```python
from build123d import *

# Parameters (mm, degrees)
SKETCH1_R           = 1.75
SKETCH1_R_2         = 1.925
BOSS_EXTRUDE1_DEPTH = 15
CUT_EXTRUDE1_DEPTH  = 8
SKETCH5_W           = 11
SKETCH5_H           = 33.5
CUT_EXTRUDE6_DEPTH  = 4
SKETCH8_R           = 1.75
CUT_EXTRUDE9_DEPTH  = 14
FILLET1_R           = 1.75
FILLET2_R           = 1
FILLET3_R           = 0.5
FILLET4_R           = 1.5


with BuildPart() as part:
    # Sketch1 → Boss-Extrude1 (new body)
    with BuildSketch(Plane.XY):
        with BuildLine():
            Line((-19, 16.75), (19, 16.75))
            Line((19, 16.75), (22.75, 16.75))
            Line((22.75, 16.75), (22.75, 13))
            ThreePointArc((22.75, 13), (22.193718688, 11.034634654), (20.689914163, 9.652360515))
            ThreePointArc((20.689914163, 9.652360515), (14.75, 0), (20.689914163, -9.652360515))
            ThreePointArc((20.689914163, -9.652360515), (22.193718688, -11.034634654), (22.75, -13))
            Line((22.75, -13), (22.75, -16.75))
            Line((22.75, -16.75), (19, -16.75))
            Line((19, -16.75), (-19, -16.75))
            Line((-19, -16.75), (-22.75, -16.75))
            Line((-22.75, -16.75), (-22.75, -13))
            ThreePointArc((-22.75, -13), (-22.193718688, -11.034634654), (-20.689914163, -9.652360515))
            ThreePointArc((-20.689914163, -9.652360515), (-14.75, 0), (-20.689914163, 9.652360515))
            ThreePointArc((-20.689914163, 9.652360515), (-22.193718688, 11.034634654), (-22.75, 13))
            Line((-22.75, 13), (-22.75, 16.75))
            Line((-22.75, 16.75), (-19, 16.75))
        make_face()
        with Locations((-10, -9.5)):
            Circle(SKETCH1_R, mode=Mode.SUBTRACT)
        with Locations((10, -9.5)):
            Circle(SKETCH1_R, mode=Mode.SUBTRACT)
        with Locations((19, 13)):
            Circle(SKETCH1_R_2, mode=Mode.SUBTRACT)
        with Locations((-19, 13)):
            Circle(SKETCH1_R_2, mode=Mode.SUBTRACT)
        with Locations((-19, -13)):
            Circle(SKETCH1_R_2, mode=Mode.SUBTRACT)
        with Locations((19, -13)):
            Circle(SKETCH1_R_2, mode=Mode.SUBTRACT)
        with Locations((-11, 0)):
            Circle(SKETCH1_R_2, mode=Mode.SUBTRACT)
        with Locations((11, 0)):
            Circle(SKETCH1_R_2, mode=Mode.SUBTRACT)
    extrude(amount=BOSS_EXTRUDE1_DEPTH)

    # Sketch2 → Cut-Extrude1 (cut)
    with BuildSketch(Plane.XY.offset(15)):
        Polygon((-4.049999999, 16.75), (-4.049999999, 14.25), (-3.149999999, 14.25), (-3.149999999, 11.25), (-4.049999999, 11.25), (-4.049999999, 8.75), (-3.149999999, 8.75), (-3.149999999, 5.75), (-4.049999999, 5.75), (-4.049999999, 3.25), (-3.149999999, 3.25), (-3.149999999, -3.25), (-4.049999999, -3.25), (-4.049999999, -5.75), (-3.149999999, -5.75), (-3.149999999, -8.75), (-4.049999999, -8.75), (-4.049999999, -11.25), (-3.149999999, -11.25), (-3.149999999, -14.25), (-4.049999999, -14.25), (-4.049999999, -16.75), (4.050000001, -16.75), (4.050000001, -14.25), (3.150000001, -14.25), (3.150000001, -11.25), (4.050000001, -11.25), (4.050000001, -8.75), (3.150000001, -8.75), (3.150000001, -5.75), (4.050000001, -5.75), (4.050000001, -3.25), (3.150000001, -3.25), (3.150000001, 3.25), (4.050000001, 3.25), (4.050000001, 5.75), (3.150000001, 5.75), (3.150000001, 8.75), (4.050000001, 8.75), (4.050000001, 11.25), (3.150000001, 11.25), (3.150000001, 14.25), (4.050000001, 14.25), (4.050000001, 16.75), align=None)
    extrude(amount=-CUT_EXTRUDE1_DEPTH, mode=Mode.SUBTRACT)

    # Sketch5 → Cut-Extrude6 (cut)
    with BuildSketch(Plane.XY.offset(15)):
        with Locations((-18.25, 0)):
            Rectangle(SKETCH5_W, SKETCH5_H)
        with Locations((18.25, 0)):
            Rectangle(SKETCH5_W, SKETCH5_H)
    extrude(amount=-CUT_EXTRUDE6_DEPTH, mode=Mode.SUBTRACT)

    # Sketch8 → Cut-Extrude9 (cut)
    with BuildSketch(Plane.XY.offset(15)):
        with Locations((7.5, 5)):
            Circle(SKETCH8_R)
        with Locations((-7.5, 5)):
            Circle(SKETCH8_R)
    extrude(amount=-CUT_EXTRUDE9_DEPTH, mode=Mode.SUBTRACT)

    # Fillet1
    # the kernel refuses this fillet: 1.75 mm, written as the material it adds along each edge
    with BuildSketch(Plane(origin=(-4.049999999, 11.25, 15), x_dir=(1, 0, 0), z_dir=(0, 0, -1)), Plane(origin=(-4.049999999, 5.75, 15), x_dir=(1, 0, 0), z_dir=(0, 0, -1)), Plane(origin=(-4.049999999, -3.25, 15), x_dir=(1, 0, 0), z_dir=(0, 0, -1)), Plane(origin=(-4.049999999, -8.75, 15), x_dir=(1, 0, 0), z_dir=(0, 0, -1)), Plane(origin=(4.050000001, -11.25, 15), x_dir=(-1, 0, 0), z_dir=(0, 0, -1))) as fillet1_piece_1:
        with BuildLine():
            CenterArc((1.75, 1.529705854), FILLET1_R, 180, 60.940718932)
            Line((0, 1.529705854), (-0.035, 1.529705854))
            Line((-0.035, 1.529705854), (-0.035, 0))
            Line((-0.035, 0), (0, -0.035))
            ThreePointArc((0, -0.035), (0.45, -0.035), (0.883, -0.030594117))
            Line((0.883, -0.030594117), (0.9, 0))
        make_face()
    extrude(amount=11.824264635)
    with BuildSketch(Plane(origin=(4.050000001, 11.25, 15), x_dir=(-1, 0, 0), z_dir=(0, 0, -1)), Plane(origin=(4.050000001, 5.75, 15), x_dir=(-1, 0, 0), z_dir=(0, 0, -1)), Plane(origin=(4.050000001, -3.25, 15), x_dir=(-1, 0, 0), z_dir=(0, 0, -1))) as fillet1_piece_2:
        with BuildLine():
            CenterArc((1.75, -1.529705854), FILLET1_R, 119.059281068, 60.940718932)
            Line((0, -1.529705854), (-0.035, -1.529705854))
            Line((-0.035, -1.529705854), (-0.035, 0))
            Line((-0.035, 0), (0, 0.035))
            ThreePointArc((0, 0.035), (0.45, 0.035), (0.883, 0.030594117))
            Line((0.883, 0.030594117), (0.9, 0))
        make_face()
    extrude(amount=11.824264635)
    with BuildSketch(Plane(origin=(4.050000001, -8.75, 15), x_dir=(0, -1, 0), z_dir=(0, 0, -1)), Plane(origin=(-4.049999999, 8.75, 15), x_dir=(0, 1, 0), z_dir=(0, 0, -1)), Plane(origin=(-4.049999999, 3.25, 15), x_dir=(0, 1, 0), z_dir=(0, 0, -1)), Plane(origin=(-4.049999999, -5.75, 15), x_dir=(0, 1, 0), z_dir=(0, 0, -1)), Plane(origin=(-4.049999999, -11.25, 15), x_dir=(0, 1, 0), z_dir=(0, 0, -1))) as fillet1_piece_3:
        with BuildLine():
            CenterArc((1.529705854, 1.75), FILLET1_R, 209.059281068, 60.940718932)
            Line((0, 0.9), (-0.030594117, 0.883))
            ThreePointArc((-0.030594117, 0.883), (-0.035, 0.45), (-0.035, 0))
            Line((-0.035, 0), (0, -0.035))
            Line((0, -0.035), (1.529705854, -0.035))
            Line((1.529705854, -0.035), (1.529705854, 0))
        make_face()
    extrude(amount=11.824264635)
    with BuildSketch(Plane(origin=(4.050000001, -5.75, 15), x_dir=(0, 1, 0), z_dir=(0, 0, -1)), Plane(origin=(4.050000001, 3.25, 15), x_dir=(0, 1, 0), z_dir=(0, 0, -1)), Plane(origin=(4.050000001, 8.75, 15), x_dir=(0, 1, 0), z_dir=(0, 0, -1))) as fillet1_piece_4:
        with BuildLine():
            CenterArc((1.529705854, -1.75), FILLET1_R, 90, 60.940718932)
            Line((0, -0.9), (-0.030594117, -0.883))
            ThreePointArc((-0.030594117, -0.883), (-0.035, -0.45), (-0.035, 0))
            Line((-0.035, 0), (0, 0.035))
            Line((0, 0.035), (1.529705854, 0.035))
            Line((1.529705854, 0.035), (1.529705854, 0))
        make_face()
    extrude(amount=11.824264635)

    # Fillet2
    fillet2_edges = [part.edges().sort_by_distance(p)[0] for p in [
        (-12.75, -16.75, 13),
        (-12.75, 16.75, 13),
        (12.75, 16.75, 13),
        (12.75, -16.75, 13),
        (-4.027502426, 10, 11),
        (-4.027502426, 4.5, 11),
        (-4.027502426, -4.5, 11),
        (-4.027502426, -10, 11),
        (4.027502428, 10, 11),
        (4.027502428, 4.5, 11),
        (4.027502428, -4.5, 11),
        (4.027502428, -10, 11),
    ]]
    fillet(fillet2_edges, radius=FILLET2_R)

    # Fillet3
    fillet3_edges = [part.edges().sort_by_distance(p)[0] for p in [
        (-4.049999999, 16.75, 11),
        (4.050000001, 16.75, 11),
        (4.050000001, -16.75, 11),
        (-4.049999999, -16.75, 11),
        (-12.75, 0.801950747, 13),
        (-12.75, -0.801950747, 13),
        (-22.75, -16.75, 5.5),
        (-22.75, 16.75, 5.5),
        (12.75, -0.801950747, 13),
        (12.75, 0.801950747, 13),
        (22.75, -16.75, 5.5),
        (22.75, 16.75, 5.5),
    ]]
    fillet(fillet3_edges, radius=FILLET3_R)

    # Fillet4
    # the kernel refuses this fillet: 1.5 mm, written as the material it adds along each edge
    with BuildSketch(Plane(origin=(-4.049999999, 14.25, 15), x_dir=(1, 0, 0), z_dir=(0, 0, -1)), Plane(origin=(4.050000001, -14.25, 15), x_dir=(-1, 0, 0), z_dir=(0, 0, -1))) as fillet4_piece_1:
        with BuildLine():
            CenterArc((1.5, -1.374772708), FILLET4_R, 113.578178478, 66.421821522)
            Line((0, -1.374772708), (-0.03, -1.374772708))
            Line((-0.03, -1.374772708), (-0.03, 0))
            Line((-0.03, 0), (0, 0.03))
            ThreePointArc((0, 0.03), (0.45, 0.03), (0.888, 0.027495454))
            Line((0.888, 0.027495454), (0.9, 0))
        make_face()
    extrude(amount=11.436931771)
    with BuildSketch(Plane(origin=(4.050000001, 14.25, 15), x_dir=(-1, 0, 0), z_dir=(0, 0, -1)), Plane(origin=(-4.049999999, -14.25, 15), x_dir=(1, 0, 0), z_dir=(0, 0, -1))) as fillet4_piece_2:
        with BuildLine():
            CenterArc((1.5, 1.374772708), FILLET4_R, 180, 66.421821522)
            Line((0, 1.374772708), (-0.03, 1.374772708))
            Line((-0.03, 1.374772708), (-0.03, 0))
            Line((-0.03, 0), (0, -0.03))
            ThreePointArc((0, -0.03), (0.45, -0.03), (0.888, -0.027495454))
            Line((0.888, -0.027495454), (0.9, 0))
        make_face()
    extrude(amount=11.436931771)


solid = part.part
```
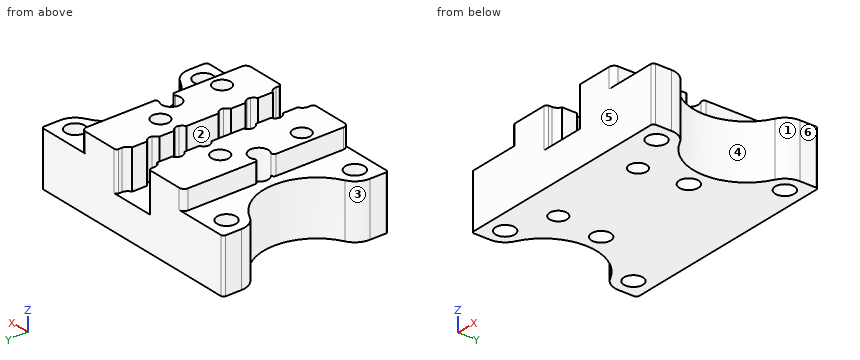
Verification items for the finished model (mm, model axes). Face numbers are marked on the shaded views. A direction names the side the tool comes from. Round coordinates to 2 decimals unless told otherwise and drop trailing zeros. Write each loop counter-clockwise with the first axis right and the second up, starting at its lowest first coordinate (ties: lowest second). Pieces come first, ordered by that corner, then holes. Notation, with made-up numbers: (-27.75, 4.5) - (-9.75, 4.5) arc R25 ccw to (-9.75, 20.5) - close; hole circle Ø3 at (-1.5, 0.25). An arc over 180 degrees is marked (long way). Answer as a JSON object with one key per item and string values. Group by question number.
Q1. Tool access check on the marked faces 1, 2 and 3. Record the directions out of +Z, -Z, +X, -X, +Y, -Y that give a thin tool (end or side, any length) a straight path to the whole face; none if there is none.
Q2. Mould release check, pull along Y, two halves, no side actions. Record for the marked faces 4, 5 and 6: released by +Y, released by -Y, zero draft, split by the parting line, or undercut.
Q3. Thickness scan on line 1 (X direction, y = -13, z = 8) (3 decimals); line 2 (X direction, y = 13, z = 1.5) (3 decimals); line 3 (X direction, y = -2, z = 11.5). Record the ranges inside material, lowest first.
Q4. Go/stop test with flat-tipped pins: pin 1 Ø1.5 at (y, z) = (7, 12.5) entering from +X; pin 2 Ø2.5 at (x, y) = (-19, -13) entering from -Z; pin 3 Ø3.5 at (y, z) = (-7, 9.5) entering from -X; pin 4 Ø3 at (x, z) = (-3, 9.5) entering from -Y. Record where each tip stops, or that it passes through.
Q5. Section check A-A, the plane z = 6. Give the number of separate pieces and of enclosed holes in the cut face, plus the area to 3 significant figures.
Q6. Section check B-B, the plane x = -11. Enter the section's corners in (y, z) (3 decimals), plus the area to 3 significant figures.
Q7. Section check D-D, the plane y = 1. Enter the section's corners in (x, z), plus the area to 3 significant figures.
Found:
{
 "1": {"face 1": "+Z, -Z, +X", "face 2": "+Z, +Y, -Y", "face 3": "+Z, -Z, -X"},
 "2": {"face 4": "undercut", "face 5": "released by -Y", "face 6": "zero draft"},
 "3": {"line 1": "x = -22.75 to -20.925, -17.075 to -3.15, 3.15 to 17.075, 20.925 to 22.75", "line 2": "x = -22.75 to -20.925, -17.075 to 17.075, 20.925 to 22.75", "line 3": "x = -12.74 to -3.15, 3.15 to 12.74"},
 "4": {"pin 1": "stops at x = 12.75", "pin 2": "passes through", "pin 3": "stops at x = -19.21", "pin 4": "stops at y = -16.75"},
 "5": {"separate pieces": "1", "enclosed holes": "10", "area": "1,160 mm^2"},
 "6": {"outline": "(-16.75, 0) - (-10.936, 0) - (-10.936, 15) - (-16.75, 15) - close; (-8.064, 0) - (-1.925, 0) - (-1.925, 15) - (-8.064, 15) - close; (1.925, 0) - (16.75, 0) - (16.75, 15) - (1.925, 15) - close", "area": "402 mm^2"},
 "7": {"outline": "(-14.8, 0) - (-12.64, 0) - (-12.64, 11) - (-14.8, 11) - close; (-9.36, 0) - (9.36, 0) - (9.36, 15) - (3.15, 15) - (3.15, 7) - (-3.15, 7) - (-3.15, 15) - (-9.36, 15) - close; (12.64, 0) - (14.8, 0) - (14.8, 11) - (12.64, 11) - close", "area": "278 mm^2"}
}
